Could you check a few things on this model? Use its own coordinates, in mm. Give positions to 0.01 mm unless a question says otherwise; leave off trailing zeros. Loops run counter-clockwise (first coordinate to the right, second up) from the corner with the lowest first, then second, coordinate; pieces in that order, holes last. Notation, with made-up numbers: (25.25, -14) - (84.25, -14) arc R30 ccw to (84.25, 12) - close; hole circle Ø8 at (-38.75, 60). An arc over 180 degrees is marked (long way). Use CSV: the item, a comma, the result in double quotes.
from build123d import *

# Parameters (mm, degrees)
F1_DEPTH = 5


with BuildPart() as f1:
    # F0 (on Top) → F1 (new body)
    with BuildSketch(Plane.XY):
        with BuildLine():
            ThreePointArc((5, 0), (1.464466, -1.464466), (0, -5))
            Line((0, -5), (0, -614.979674))
            ThreePointArc((0, -614.979674), (1.478868, -618.529551), (5.04065, -619.979509))
            ThreePointArc((5.04065, -619.979509), (128.100613, -606.621985), (246.054486, -569.084519))
            ThreePointArc((246.054486, -569.084519), (248.567798, -566.67948), (248.90409, -563.217131))
            Line((248.90409, -563.217131), (100.984028, -3.722003))
            ThreePointArc((100.984028, -3.722003), (99.200525, -1.03831), (96.150114, 0))
            Line((96.150114, 0), (5, 0))
        make_face()
    extrude(amount=F1_DEPTH)


solid = f1.part
1) I'm going to push a flat-ended pin straight in: P1, Ø3, axis at x = 126.5, z = 2.5, coming from the -Y side. Where does the tip first touch, or does it pass through?
Answer below:
P1,"stops at y = -607.27"
2) Suppose I cut it at B-B (x = 146). Please give me the cut outline in (y, z), plus the area to 3 significant figures.
Answer below:
outline,"(-602.56, 0) - (-173.99, 0) - (-173.99, 5) - (-602.56, 5) - close"
area,"2,140 mm2"
3) I need wall thicknesses on line 1 along X through (y, z) = (-361, 3); line 2 along Y through (x, z) = (83, 3.15); line 3 along Y through (x, z) = (85, 1.8). Which ranges of each line are inside material? Lowest first, please.
Answer below:
line 1,"x = 0 to 195.44"
line 2,"y = -614.42 to 0"
line 3,"y = -614.15 to 0"
4) Suppose I cut it at C-C (y = -240.5). Please give me the cut outline in (x, z), plus the area to 3 significant figures.
Answer below:
outline,"(0, 0) - (163.58, 0) - (163.58, 5) - (0, 5) - close"
area,"818 mm2"
5) Suppose I cut it at A-A (z = 3.85). Please give me the cut outline in (x, y), plus the area to 3 significant figures.
Answer below:
outline,"(0, -614.98) arc R5 ccw to (5.04, -619.98) arc R620 ccw to (246.05, -569.08) arc R5 ccw to (248.9, -563.22) - (100.98, -3.72) arc R5 ccw to (96.15, 0) - (5, 0) arc R5 ccw to (0, -5) - close"
area,"108,000 mm2"
